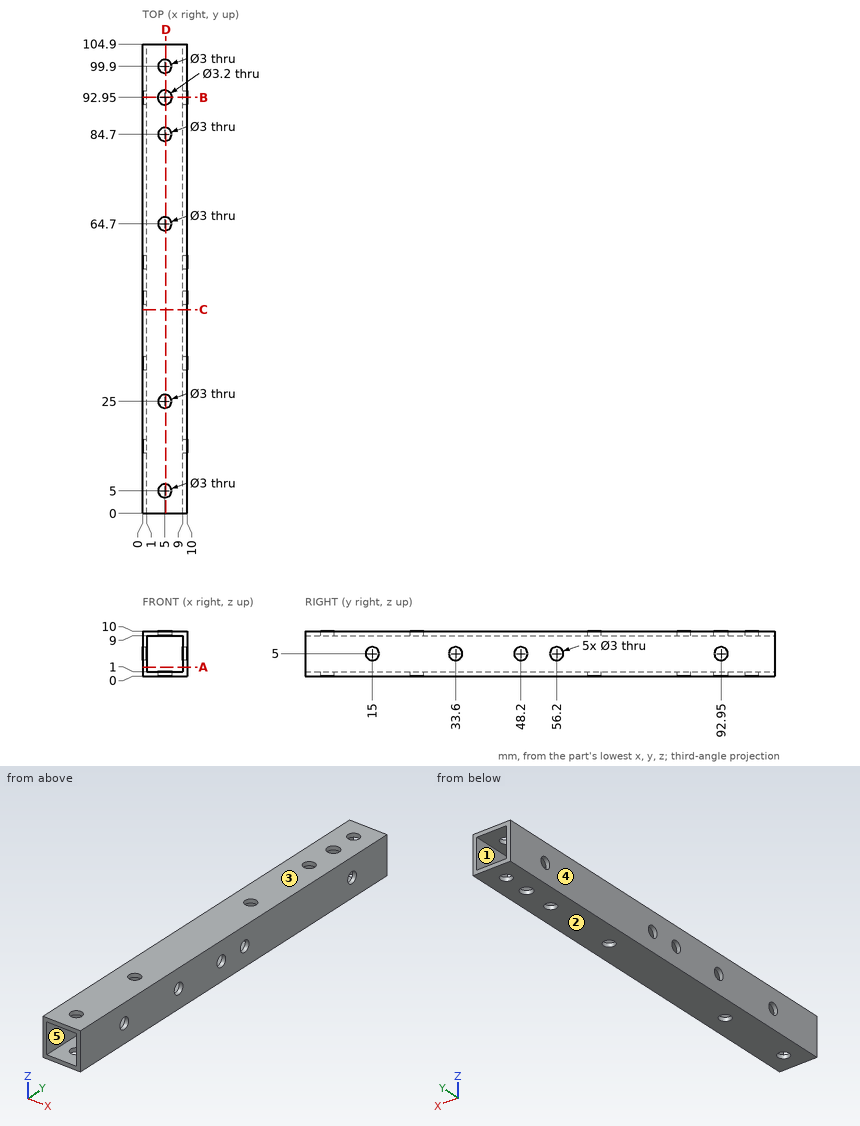
Can you work these out from the drawing? Everything is in mm from the part's minimum corner. A direction names the side the tool comes from. Coordinates: 2 decimals unless noted, no trailing zeros. Loops run counter-clockwise (first coordinate to the right, second up) from the corner with the lowest first, then second, coordinate; pieces in that order, holes last. Notation, with made-up numbers: (87, -15) - (134, -15) arc R19 cw to (134, 15) - close; hole circle Ø2 at (60.5, -35). An arc over 180 degrees is marked (long way). Put each result on its own line as item: value. Start each with the question number.
Item 1: If I drill on line 1 along X through (y, z) = (86.5, 6.75); line 2 along Y through (x, z) = (9.35, 5); line 3 along X through (y, z) = (64.7, 9.45), over which ranges is the centre line in solid material (lowest first)?
Item 2: For pin 1 (2.5 mm diameter, centred on x = 5, y = 25, fed in from -Z), with a flat end and sliding along its axis, tell me the tip position at first contact or that it passes through.
Item 3: Suppose I cut it at B-B (y = 92.95). Please give me the cut outline in (x, z), and give its area (3 significant figures).
Item 4: Suppose I cut it at C-C (y = 45.5). Please give me the cut outline in (x, z).
Item 5: Which directions (+Z, -Z, +X, -X, +Y, -Y) give clear straight access to the entire face, cutting with the end or side of a thin tool? Please do the marked faces 1 and 2.
Item 6: Suppose I cut it at A-A (z = 2). Please give me the cut outline in (x, y).
Item 7: Suppose I cut it at D-D (x = 5.25). State how many separate pieces and enclosed holes the cut face has, and give its area (3 significant figures).
Item 8: If we mould it in two halves opening along Z, with no side actions, what happens to the marked faces 3, 4 and 5? For each: +Z half, -Z half, draft (parallel to the pull), parting line (faces both ways), or undercut.
Here are the results:
1. line 1: 0 to 1, 9 to 10
1. line 2: 0 to 13.5, 16.5 to 32.1, 35.1 to 46.7, 49.7 to 54.7, 57.7 to 91.45, 94.45 to 104.9
1. line 3: 0 to 3.5, 6.5 to 10
2. pin 1: through
3. outline: (0, 0) - (3.4, 0) - (3.4, 1) - (1, 1) - (1, 3.5) - (0, 3.5) - close; (0, 6.5) - (1, 6.5) - (1, 9) - (3.4, 9) - (3.4, 10) - (0, 10) - close; (6.6, 0) - (10, 0) - (10, 3.5) - (9, 3.5) - (9, 1) - (6.6, 1) - close; (6.6, 9) - (9, 9) - (9, 6.5) - (10, 6.5) - (10, 10) - (6.6, 10) - close
3. area: 23.6 mm²
4. outline: (0, 0) - (10, 0) - (10, 10) - (0, 10) - close; hole (1, 1) - (9, 1) - (9, 9) - (1, 9) - close
5. face 1: +Y, -Y
5. face 2: -Z, +X, -X, +Y, -Y
6. outline: (0, 0) - (1, 0) - (1, 104.9) - (0, 104.9) - close; (9, 0) - (10, 0) - (10, 104.9) - (9, 104.9) - close
7. separate pieces: 14
7. enclosed holes: 0
7. area: 174 mm²
8. face 3: +Z half
8. face 4: draft
8. face 5: undercut
